from build123d import *

# Parameters (mm, degrees)
BOSS_EXTRUDE1_DEPTH  = 1.5
BOSS_EXTRUDE2_START  = 1.5
SKETCH1_3_W          = 6.5
SKETCH1_3_H          = 7.4
SKETCH1_3_W_2        = 1.6
SKETCH1_3_H_2        = 2.3
BOSS_EXTRUDE2_DEPTH  = 4
CUT_EXTRUDE1_DEPTH   = 5.5
MIRROR2_COPY_1_DEPTH = 5.5
CUT_EXTRUDE2_DEPTH   = 4
SKETCH6_W            = 1.613740729
SKETCH6_H            = 4.851761748
BOSS_EXTRUDE3_DEPTH  = 2


with BuildPart() as part:
    # Sketch1 → Boss-Extrude1 (new body)
    with BuildSketch(Plane.XY):
        Polygon((6.974355653, -28), (31.223066959, -14), (31.223066959, 14), (6.974355653, 28), (-41.523066959, 14), (-41.523066959, -14), align=None)
    extrude(amount=BOSS_EXTRUDE1_DEPTH)

    # Sketch1<3> → Boss-Extrude2 (add)
    with BuildSketch(Plane.XY.offset(BOSS_EXTRUDE2_START)):
        Polygon((6.974355653, 28), (-41.523066959, 14), (-41.523066959, -14), (6.974355653, -28), (31.223066959, -14), (31.223066959, 14), align=None)
        with Locations((-5.15, 0)):
            Rectangle(SKETCH1_3_W, SKETCH1_3_H, mode=Mode.SUBTRACT)
        with Locations((-39.123066959, -2.55)):
            Rectangle(SKETCH1_3_W_2, SKETCH1_3_H_2, mode=Mode.SUBTRACT)
        with Locations((-39.123066959, 2.55)):
            Rectangle(SKETCH1_3_W_2, SKETCH1_3_H_2, mode=Mode.SUBTRACT)
    extrude(amount=BOSS_EXTRUDE2_DEPTH)

    # WireCutExtrude → Cut-Extrude1 (cut)
    with BuildSketch(Plane.XY.offset(5.5)):
        Polygon((-9.094946311, 10.972481296), (-10.538213003, 5.388213003), (-16.122481296, 3.944946311), (-16.873171174, 6.849505608), (-13.000425446, 7.850425446), (-11.999505608, 11.723171174), align=None)
    cut_extrude1 = extrude(amount=-CUT_EXTRUDE1_DEPTH, mode=Mode.SUBTRACT)

    # Mirror1: Cut-Extrude1 across plane
    add(cut_extrude1.mirror(Plane(origin=(0, 0, 0), x_dir=(0, 0, 1), z_dir=(0, -1, 0))), mode=Mode.SUBTRACT)

    # Mirror2: Cut-Extrude1 across plane
    add(cut_extrude1.mirror(Plane(origin=(-5.15, 0, 0), x_dir=(0, 0, 1), z_dir=(1, 0, 0))), mode=Mode.SUBTRACT)

    # Mirror2 copy 1 sketch → Mirror2 copy 1 (cut)
    with BuildSketch(Plane(origin=(-10.3, 0, 5.5), x_dir=(-1, 0, 0), z_dir=(0, 0, 1))):
        Polygon((-9.094946311, 10.972481296), (-10.538213003, 5.388213003), (-16.122481296, 3.944946311), (-16.873171174, 6.849505608), (-13.000425446, 7.850425446), (-11.999505608, 11.723171174), align=None)
    extrude(amount=-MIRROR2_COPY_1_DEPTH, mode=Mode.SUBTRACT)

    # Sketch5 → Cut-Extrude2 (cut)
    with BuildSketch(Plane.XY.offset(5.5)):
        Polygon((-10.264722381, 6.44639928), (-6.786259271, 3.7), (-8.4, 3.7), (-8.4, 2.425880874), (-11.753980013, 5.073995286), (-10.538213003, 5.388213003), align=None)
        Polygon((-3.513740729, 3.7), (-0.035277619, 6.44639928), (0.238213003, 5.388213003), (1.453980013, 5.073995286), (-1.9, 2.425880874), (-1.9, 3.7), align=None)
        Polygon((-36.823066959, 1.4), (-36.823066959, 3.7), (-16.873171174, 6.849505608), (-16.122481296, 3.944946311), align=None)
    cut_extrude2 = extrude(amount=-CUT_EXTRUDE2_DEPTH, mode=Mode.SUBTRACT)

    # Mirror3: Cut-Extrude2 across plane
    add(cut_extrude2.mirror(Plane(origin=(0, 0, 0), x_dir=(0, 0, 1), z_dir=(0, -1, 0))), mode=Mode.SUBTRACT)

    # Sketch6 → Boss-Extrude3 (add)
    with BuildSketch(Plane.XY.offset(1.5)):
        with Locations((-2.706870365, 0)):
            Rectangle(SKETCH6_W, SKETCH6_H)
        with Locations((-7.593129636, 0)):
            Rectangle(SKETCH6_W, SKETCH6_H)
    extrude(amount=BOSS_EXTRUDE3_DEPTH)


solid = part.part
Work out the finished part from the listing and answer in its coordinate system (mm). A direction names the side the tool comes from. Give positions to 0.01 mm unless a question says otherwise; leave off trailing zeros. Order: outer loops, then holes, each group sorted by start corner. A loop starts at its lowest first (then second) coordinate and runs counter-clockwise, first axis right, second up. Notation, with made-up numbers: (-28, 75) -> (9, 75) arc R21 ccw to (9, 89) -> close; hole circle Ø11 at (23, -25.75). An arc over 180 degrees is marked (long way). One line per item, written item: value.
Item 1: Find section B-B, the plane z = 2.75. State how many separate pieces and enclosed holes the cut face has, plus the area to 3 significant figures.
Answer sheet:
separate pieces: 1
enclosed holes: 3
area: 2,760 mm²
Item 2: Find section D-D, the plane y = -17. Give the vertices of the cut face in (x, z), plus the area to 3 significant figures.
Answer sheet:
outline: (-31.13, 0) -> (26.03, 0) -> (26.03, 5.5) -> (-31.13, 5.5) -> close
area: 314 mm²
Item 3: Find section C-C, the plane x = -5. Give the vertices of the cut face in (y, z).
Answer sheet:
outline: (-24.54, 0) -> (24.54, 0) -> (24.54, 5.5) -> (3.7, 5.5) -> (3.7, 1.5) -> (-3.7, 1.5) -> (-3.7, 5.5) -> (-24.54, 5.5) -> close
Item 4: A tool of negligible diameter and unlimited length cuts with its end or side. For faces 4 (the flat face through (-9.646, -8.84, 2.788)), 5 (the flat face through (18.929, -21.098, 2.712)), 6 (the flat face through (-3.514, 0, 2)), from which of +Z, -Z, +X, -X, +Y, -Y can it reach the whole face along a straight path? Write none if from no direction.
Answer sheet:
face 4: +Z, -Z
face 5: +Z, -Z, +X, -Y
face 6: +Z
Item 5: Find section A-A, the plane x = -14.5. Give the vertices of the cut face in (y, z), plus the area to 3 significant figures.
Answer sheet:
outline: (-21.8, 0) -> (-7.46, 0) -> (-7.46, 5.5) -> (-21.8, 5.5) -> close; (-4.36, 0) -> (4.36, 0) -> (4.36, 5.5) -> (-4.36, 5.5) -> close; (7.46, 0) -> (21.8, 0) -> (21.8, 5.5) -> (7.46, 5.5) -> close
area: 206 mm²
Item 6: Straight lines are drawn through the part: probe 1 along Y at (x, z) = (-35, 1.8); probe 2 along X at (y, z) = (-1, 1.55); probe 3 along Y at (x, z) = (3, 2.1). For each, find the intervals that lie inside material, in ascending order.
Answer sheet:
probe 1: -15.88 to -3.99, -1.62 to 1.62, 3.99 to 15.88
probe 2: -41.52 to -6.79, -3.51 to 31.22
probe 3: -26.85 to -7.77, -4.67 to 4.67, 7.77 to 26.85
Item 7: Flat-ended cylindrical pins translate along their axes: P1, Ø1.8, axis at x = -7.5, z = 2.5, coming from the -Y side; P2, Ø1.8, axis at x = -39, z = 3.5, coming from the +Y side; P3, Ø6.5, axis at x = -4.5, y = -1, coming from the +Z side; P4, Ø0.8, axis at x = -2.5, y = -1, coming from the +Z side. Find the tip coordinate at first contact, or state that the pin passes through.
Answer sheet:
P1: y = -24.08
P2: y = 14.99
P3: z = 5.5
P4: z = 3.5
Item 8: Determine the mould class of faces 1 (the flat face through (-16.93, 21.1, 2.71)), 2 (the flat face through (31.223, 0, 3)), 3 (the flat face through (-1.799, 5.054, 3.528)) for opening direction Y: released by +Y, released by -Y, zero draft, split by the parting line, or undercut.
Answer sheet:
face 1: released by +Y
face 2: zero draft
face 3: undercut
